Design review of the part shown in the three views and the two pictorial views. Dimensions are in mm from the part's minimum x, y and z. Round coordinates to 2 decimals unless told otherwise and drop trailing zeros. Loops run counter-clockwise (first coordinate to the right, second up) from the corner with the lowest first, then second, coordinate; pieces in that order, holes last. Notation, with made-up numbers: M 26,-36.75 L 35,-36.75 A32 cw 35,-2.75 Z; hole C 33.25,16.5 d9. An arc over 180 degrees is marked long. One line per question, with ' | ' between items. Start each with the question number.
1) We need section C-C (x = 23). Give the boundary of the cut face in (y, z), and give its area (3 significant figures).
2) For pin 1 Ø2 at (y, z) = (6.5, 2.5) entering from +X; pin 2 Ø0.6 at (x, y) = (1, 4.5) entering from +Z; pin 3 Ø0.6 at (y, z) = (6.5, 3) entering from +X; pin 4 Ø0.6 at (y, z) = (5.5, 3) entering from -X, all flat-tipped, find the tip position at first contact; note any pin that passes through.
3) We need section D-D (z = 0.55). Give the boundary of the cut face in (x, y).
4) We need section A-A (y = 13.75). Give the boundary of the cut face in (x, z), and give its area (3 significant figures).
5) For probe 1 along X at (y, z) = (9.5, 3.45); probe 2 along X at (y, z) = (1, 1.35); probe 3 along X at (y, z) = (1, 2.1), list the stretches that pass through material, from the lowest coordinate up. Write a range as from..to.
6) We need section B-B (z = 3.4). Give the boundary of the cut face in (x, y).
7) Mouldability with a two-part tool opening along X and no side actions: class the marked faces 1 and 2 as pulls with the +X half, pulls with the -X half, needs draft (parallel to the pull), parting line crosses it, or undercut.
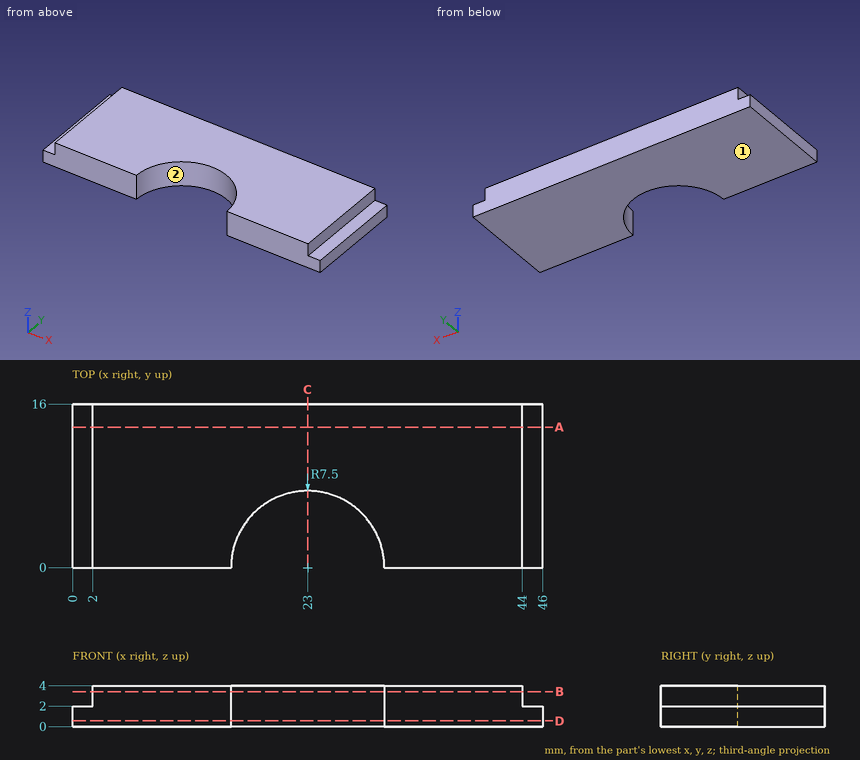
Answers below:
1) outline: M 7.5,0 L 16,0 L 16,4 L 7.5,4 Z | area: 34.0 mm^2
2) pin 1: x = 46 | pin 2: z = 2 | pin 3: x = 44 | pin 4: x = 2
3) outline: M 0,0 L 15.5,0 A7.5 cw 30.5,0 L 46,0 L 46,16 L 0,16 Z
4) outline: M 0,0 L 46,0 L 46,2 L 44,2 L 44,4 L 2,4 L 2,2 L 0,2 Z | area: 176 mm^2
5) probe 1: 2..44 | probe 2: 0..15.57, 30.43..46 | probe 3: 2..15.57, 30.43..44
6) outline: M 2,0 L 15.5,0 A7.5 cw 30.5,0 L 44,0 L 44,16 L 2,16 Z
7) face 1: needs draft | face 2: undercut
